Check sheet for the modelled part. Datum: model origin and axes. Units: mm. A direction names the side the tool comes from. Round coordinates to 2 decimals unless told otherwise and drop trailing zeros. Order: outer loops, then holes, each group sorted by start corner. A loop starts at its lowest first (then second) coordinate and runs counter-clockwise, first axis right, second up. Notation, with made-up numbers: (88.25, -34.75) -> (113.25, -34.75) arc R25 ccw to (113.25, -18.75) -> close; hole circle Ø10 at (7, 28.5). An arc over 180 degrees is marked (long way). Answer in a Markdown table with one row per item.
from build123d import *

# Parameters (mm, degrees)
F0_W          = 12.446
F0_H          = 12.446
F1_DEPTH      = 7.62
F2_R          = 7.62
F3_DEPTH      = 35.56
F4_R          = 2.54
F5_DEPTH      = 7.62
F5_DEPTH_BACK = 25.4


with BuildPart() as f1:
    # F0 (on Front) → F1 (new body)
    with BuildSketch(Plane.XZ):
        with Locations((-31.3575975597, 36.4074829547)):
            Rectangle(F0_W, F0_H)
    extrude(amount=F1_DEPTH)

    # F2 (on face) → F3 (join)
    with BuildSketch(Plane.XZ.offset(7.62)):
        with Locations((-31.3575975597, 36.4074829547)):
            Circle(F2_R)
    extrude(amount=F3_DEPTH)

    # F4 (on face) → F5 (cut, two sides)
    with BuildSketch(Plane.XY.offset(42.6304829547)) as f5_sk:
        with Locations((-31.3575975597, -17.78)):
            Circle(F4_R)
        with Locations((-31.3575975597, -27.94)):
            Circle(F4_R)
        with Locations((-31.3575975597, -38.1)):
            Circle(F4_R)
    extrude(amount=-F5_DEPTH, mode=Mode.SUBTRACT)
    extrude(f5_sk.sketch, amount=F5_DEPTH_BACK, mode=Mode.SUBTRACT)


solid = f1.part
Item 1: Depth check by flat-ended pin: P1, Ø6, axis at y = -11.5, z = 30.5, coming from the +X side; P2, Ø1.5, axis at x = -30.5, y = -38, coming from the +Z side; P3, Ø4, axis at x = -32.5, y = -5.5, coming from the -Z side. Enter the tip coordinate at first touch or a pass-through.
Result sheet:
| item | result |
|---|---|
| P1 | stops at x = -24.31 |
| P2 | stops at z = 35.01 |
| P3 | stops at z = 30.18 |
Item 2: Mould release check, pull along Y, two halves, no side actions. Record for faces 1 (the cylindrical face through (-33, -26, 39)), 2 (the flat face through (-37, -7.62, 31)), 3 (the flat face through (-31, -4, 42.63)): pulls with the +Y half, pulls with the -Y half, needs draft (parallel to the pull), parting line crosses it, or undercut.
Result sheet:
| item | result |
|---|---|
| face 1 | undercut |
| face 2 | pulls with the -Y half |
| face 3 | needs draft |
Item 3: Cross-section at A-A (x = -31). Record the boundary of the cut face in (y, z).
Result sheet:
| item | result |
|---|---|
| outline | (-43.18, 28.8) -> (-7.62, 28.8) -> (-7.62, 30.18) -> (0, 30.18) -> (0, 42.63) -> (-7.62, 42.63) -> (-7.62, 44.02) -> (-15.27, 44.02) -> (-15.27, 35.01) -> (-20.29, 35.01) -> (-20.29, 44.02) -> (-25.43, 44.02) -> (-25.43, 35.01) -> (-30.45, 35.01) -> (-30.45, 44.02) -> (-35.59, 44.02) -> (-35.59, 35.01) -> (-40.61, 35.01) -> (-40.61, 44.02) -> (-43.18, 44.02) -> close |
Item 4: Cross-section at D-D (x = -36.75). Record the boundary of the cut face in (y, z), and give its area (3 significant figures).
Result sheet:
| item | result |
|---|---|
| outline | (-43.18, 31.02) -> (-7.62, 31.02) -> (-7.62, 30.18) -> (0, 30.18) -> (0, 42.63) -> (-7.62, 42.63) -> (-7.62, 41.79) -> (-43.18, 41.79) -> close |
| area | 478 mm^2 |
Item 5: Scan lines: line 1 (Y direction, x = -32.5, z = 40); line 2 (Y direction, x = -32, z = 36.25); line 3 (X direction, y = -4, z = 39). Record each from-to range of solid material in increasing order. Write a range as [from, to].
Result sheet:
| item | result |
|---|---|
| line 1 | y = [-43.18, -40.37], [-35.83, -30.21], [-25.67, -20.05], [-15.51, 0] |
| line 2 | y = [-43.18, -40.56], [-35.64, -30.4], [-25.48, -20.24], [-15.32, 0] |
| line 3 | x = [-37.58, -25.13] |
Item 6: Cross-section at C-C (z = 31.25). Record the boundary of the cut face in (x, y), and give its area (3 significant figures).
Result sheet:
| item | result |
|---|---|
| outline | (-37.58, -7.62) -> (-36.97, -7.62) -> (-36.97, -43.18) -> (-25.75, -43.18) -> (-25.75, -7.62) -> (-25.13, -7.62) -> (-25.13, 0) -> (-37.58, 0) -> close |
| area | 494 mm^2 |
Item 7: Cross-section at B-B (y = -3.5). Record the boundary of the cut face in (x, z), and give its area (3 significant figures).
Result sheet:
| item | result |
|---|---|
| outline | (-37.58, 30.18) -> (-25.13, 30.18) -> (-25.13, 42.63) -> (-37.58, 42.63) -> close |
| area | 155 mm^2 |
Item 8: Set-up check for faces 4 (the cylindrical face through (-33.23, -16.063, 39.457)), 5 (the flat face through (-25.7, -7.62, 30.7)), 6 (the flat face through (-37, -7.62, 42)), 7 (the flat face through (-25.135, -4, 36)), 8 (the flat face through (-25.7, -7.62, 42.1)): record each of +Z, -Z, +X, -X, +Y, -Y from which the full face is reachable in a straight line by a thin tool's end or side.
Result sheet:
| item | result |
|---|---|
| face 4 | +Z |
| face 5 | -Z, +X, -Y |
| face 6 | +Z, -X, -Y |
| face 7 | +Z, -Z, +X, +Y |
| face 8 | +Z, +X, -Y |
